Source: three-view drawing plus pictorial views. Frame: mm from the lowest corner of the part. A direction names the side the tool comes from. Coordinates: 2 decimals unless noted, no trailing zeros. Loops run counter-clockwise (first coordinate to the right, second up) from the corner with the lowest first, then second, coordinate; pieces in that order, holes last. Notation, with made-up numbers: M 16,-39 L 71,-39 A24 cw 71,-21 Z; hole C 1.5,51 d9. An arc over 180 degrees is marked long. Use a Markdown table: item, result. Add a question column.
1. Pin query (flat end, axial travel): pin 1 (1.5 mm diameter, centred on x = 8.5, z = 0.5, fed in from -Y); pin 2 (0.8 mm diameter, centred on x = 5, z = 1.5, fed in from -Y); pin 3 (1 mm diameter, centred on x = 10, y = 14, fed in from -Z); pin 4 (1.5 mm diameter, centred on y = 6.5, z = 1, fed in from -X). Return the tip coordinate at first contact, or that it passes through.
2. Set-up query: the marked faces 4 and 5. Return all of +Z, -Z, +X, -X, +Y, -Y with unobstructed straight access to the full face (end or side cutting, diameter ignored); none if empty.
3. Section A-A on y = 14. Output: boundary loops of the cut face in (x, z), then the cut area to 3 significant figures.
4. Line query: L1, parallel to Y at x = 10.5, z = 0.7; L2, parallel to Y at x = 11.75, z = 0.55; L3, parallel to X at y = 4.5, z = 2.15. Output: solid intervals per line, ascending. Write a range as [from, to].
5. Section C-C on y = 3.5. Output: boundary loops of the cut face in (x, z), then the cut area to 3 significant figures.
6. Draft query along X for the marked faces 1, 2 and 3. Return one class per face: +X half, -X half, draft (parallel to the pull), parting line (faces both ways), or undercut.
7. Section D-D on x = 1.75. Output: boundary loops of the cut face in (y, z), then the cut area to 3 significant figures.
8. Section B-B on z = 1.4. Output: boundary loops of the cut face in (x, y), then the cut area to 3 significant figures.
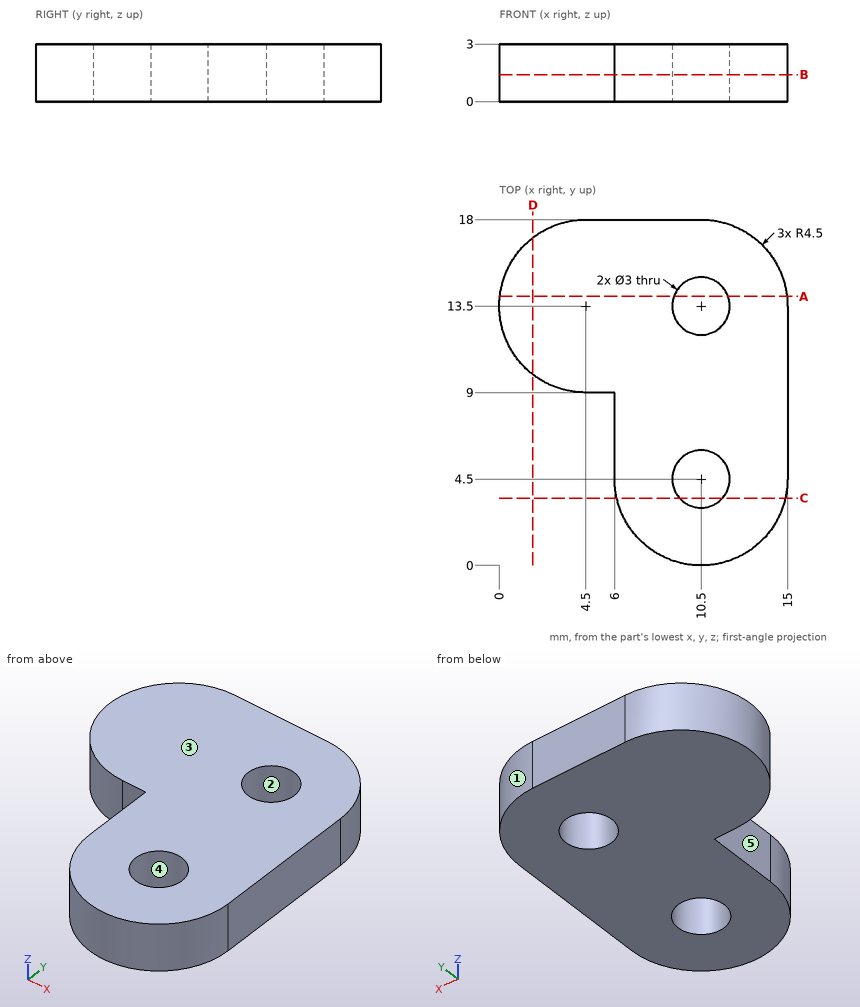
Answers below:
| question | item | result |
|---|---|---|
| 1 | pin 1 | stops at y = 0.18 |
| 1 | pin 2 | stops at y = 9 |
| 1 | pin 3 | passes through |
| 1 | pin 4 | stops at x = 6 |
| 2 | face 4 | +Z, -Z |
| 2 | face 5 | +Z, -Z, -X, -Y |
| 3 | outline | M 0.03,0 L 9.09,0 L 9.09,3 L 0.03,3 Z; M 11.91,0 L 14.97,0 L 14.97,3 L 11.91,3 Z |
| 3 | area | 36.3 mm² |
| 4 | L1 | y = [0, 3], [6, 12], [15, 18] |
| 4 | L2 | y = [0.18, 3.67], [5.33, 12.67], [14.33, 17.82] |
| 4 | L3 | x = [6, 9], [12, 15] |
| 5 | outline | M 6.11,0 L 9.38,0 L 9.38,3 L 6.11,3 Z; M 11.62,0 L 14.89,0 L 14.89,3 L 11.62,3 Z |
| 5 | area | 19.6 mm² |
| 6 | face 1 | +X half |
| 6 | face 2 | undercut |
| 6 | face 3 | draft |
| 7 | outline | M 9.94,0 L 17.06,0 L 17.06,3 L 9.94,3 Z |
| 7 | area | 21.4 mm² |
| 8 | outline | M 4.5,9 L 6,9 L 6,4.5 A4.5 ccw 15,4.5 L 15,13.5 A4.5 ccw 10.5,18 L 4.5,18 A4.5 ccw Z; hole C 10.5,4.5 d3; hole C 10.5,13.5 d3 |
| 8 | area | 180 mm² |
